from build123d import *

# Parameters (mm, degrees)
F1_DEPTH = 8.5


# Not quite as in the source:
# - a feature names something its author has since deleted; it is built from what else it names


with BuildPart() as f1:
    # F0 (on Top) → F1 (new body)
    with BuildSketch(Plane.XY):
        with BuildLine():
            ThreePointArc((-9.25, -7.6444424257), (-11.6891485981, -2.7136331829), (-11.6717637121, 2.7874597484))
            ThreePointArc((-11.6717637121, 2.7874597484), (-11.2656904289, 4.1333060811), (-10.7050113586, 5.42242859))
            Line((-10.7050113586, 5.42242859), (-5.8459149373, 18.8072078091))
            ThreePointArc((-5.8459149373, 18.8072078091), (0, 22.4041745059), (5.8459149373, 18.8072078091))
            Line((5.8459149373, 18.8072078091), (10.7050113586, 5.42242859))
            ThreePointArc((10.7050113586, 5.42242859), (11.2656904289, 4.1333060811), (11.6717637121, 2.7874597484))
            ThreePointArc((11.6717637121, 2.7874597484), (11.6891485981, -2.7136331829), (9.25, -7.6444424257))
            Line((9.25, -7.6444424257), (9.25, -11.1663557171))
            Line((9.25, -11.1663557171), (9.25, -20.1444424257))
            Line((9.25, -20.1444424257), (3.25, -20.1444424257))
            Line((3.25, -20.1444424257), (3.25, -21.1444424257))
            Line((3.25, -21.1444424257), (3.25, -23.6444424257))
            Line((3.25, -23.6444424257), (7, -26.1444424257))
            Line((7, -26.1444424257), (9.25, -26.1444424257))
            Line((9.25, -26.1444424257), (9.25, -27.6444424257))
            Line((9.25, -27.6444424257), (14.25, -27.6444424257))
            Line((14.25, -27.6444424257), (14.25, -21.4303609628))
            Line((14.25, -21.4303609628), (14.25, -2.6809513237))
            ThreePointArc((14.25, -2.6809513237), (14.437364718, -1.3462912018), (14.5, 0))
            ThreePointArc((14.5, 0), (14.400503927, 1.6957259941), (14.1033811521, 3.3681805293))
            ThreePointArc((14.1033811521, 3.3681805293), (13.8091695526, 4.4223111907), (13.4362898945, 5.4512488358))
            Line((13.4362898945, 5.4512488358), (8.4985279846, 18.8072078091))
            ThreePointArc((8.4985279846, 18.8072078091), (0, 24.7259901099), (-8.4985279846, 18.8072078091))
            Line((-8.4985279846, 18.8072078091), (-13.4362898945, 5.4512488358))
            ThreePointArc((-13.4362898945, 5.4512488358), (-13.8091695526, 4.4223111907), (-14.1033811521, 3.3681805293))
            ThreePointArc((-14.1033811521, 3.3681805293), (-14.400503927, 1.6957259941), (-14.5, 0))
            ThreePointArc((-14.5, 0), (-14.437364718, -1.3462912018), (-14.25, -2.6809513237))
            Line((-14.25, -2.6809513237), (-14.25, -21.1444424257))
            Line((-14.25, -21.1444424257), (-14.25, -27.6444424257))
            Line((-14.25, -27.6444424257), (-9.25, -27.6444424257))
            Line((-9.25, -27.6444424257), (-9.25, -26.1444424257))
            Line((-9.25, -26.1444424257), (-7, -26.1444424257))
            Line((-7, -26.1444424257), (-3.25, -23.6444424257))
            Line((-3.25, -23.6444424257), (-3.25, -21.1444424257))
            Line((-3.25, -21.1444424257), (-3.25, -20.1444424257))
            Line((-3.25, -20.1444424257), (-9.25, -20.1444424257))
            Line((-9.25, -20.1444424257), (-9.25, -11.1663557171))
            Line((-9.25, -11.1663557171), (-9.25, -7.6444424257))
        make_face()
    extrude(amount=-F1_DEPTH)


solid = f1.part
Verification items for the finished model (mm, model axes). A direction names the side the tool comes from. Give positions to 0.01 mm unless a question says otherwise; leave off trailing zeros. Order: outer loops, then holes, each group sorted by start corner. A loop starts at its lowest first (then second) coordinate and runs counter-clockwise, first axis right, second up. Notation, with made-up numbers: M 5.5,78 L 9.5,78 A21 cw 9.5,99 Z; hole C 82,7.5 d8. An arc over 180 degrees is marked long. Use one line per item in the form item = value. Start each with the question number.
Q1. Section check C-C (x = -4). Enter the section's corners in (y, z).
Q2. Mould release check, pull along X, two halves, no side actions. Record for faces 4 (the cylindrical face through (0.154, 24.725, -4.19)), 5 (the flat face through (14.25, -15, -4)), 6 (the flat face through (5.1, -24.88, -4.19)): +X half, -X half, draft (parallel to the pull), parting line (faces both ways), or undercut.
Q3. Scan lines: line 1 along X through (y, z) = (-14, -4.25); line 2 along X through (y, z) = (-23.5, -7.25); line 3 along Y through (x, z) = (4, -4.25). Record each from-to range of solid material in increasing order. Write a range as [from, to].
Q4. Section check A-A (y = -12.5). Enter the section's corners in (x, z), then the cut area to 3 significant figures.
Q5. Access from +Z, -Z, +X, -X, +Y, -Y to the whole of each face (thin tool, end or side, straight path). Record for faces 1 (the flat face through (-14.25, -15, -4)), 2 (the flat face through (-9.25, -14, -4)), 3 (the flat face through (-8, -26.144, -4)).
Q6. Section check B-B (z = -7). Enter the section's corners in (x, y).
Q7. Go/stop test with flat-tipped pins: pin 1 Ø4 at (y, z) = (-21.5, -5) entering from -X; pin 2 Ø5 at (x, z) = (-5, -3.5) entering from +Y; pin 3 Ø1 at (x, z) = (-1, -5) entering from +Y; pin 4 Ø6 at (x, y) = (6.5, -18.5) entering from +Z. Record where each tip stops, or that it passes through.
Q8. Section check D-D (x = -0.75). Enter the section's corners in (y, z), then the cut area to 3 significant figures.
Evaluation:
q1.outline = M -24.14,-8.5 L -20.14,-8.5 L -20.14,0 L -24.14,0 Z; M 21.04,-8.5 L 23.8,-8.5 L 23.8,0 L 21.04,0 Z
q2.face_4 = parting line
q2.face_5 = +X half
q2.face_6 = undercut
q3.line_1 = [-14.25, -9.25], [9.25, 14.25]
q3.line_2 = [-14.25, -3.25], [3.25, 14.25]
q3.line_3 = [-24.14, -20.14], [21.04, 23.8]
q4.outline = M -14.25,-8.5 L -9.25,-8.5 L -9.25,0 L -14.25,0 Z; M 9.25,-8.5 L 14.25,-8.5 L 14.25,0 L 9.25,0 Z
q4.area = 85.0 mm2
q5.face_1 = +Z, -Z, -X, -Y
q5.face_2 = +Z, -Z
q5.face_3 = +Z, -Z, -Y
q6.outline = M -14.25,-27.64 L -9.25,-27.64 L -9.25,-26.14 L -7,-26.14 L -3.25,-23.64 L -3.25,-20.14 L -9.25,-20.14 L -9.25,-7.64 A12 cw -10.71,5.42 L -5.85,18.81 A6.55 cw 5.85,18.81 L 10.71,5.42 A12 cw 9.25,-7.64 L 9.25,-20.14 L 3.25,-20.14 L 3.25,-23.64 L 7,-26.14 L 9.25,-26.14 L 9.25,-27.64 L 14.25,-27.64 L 14.25,-2.68 A14.5 ccw 13.44,5.45 L 8.5,18.81 A9.06 ccw -8.5,18.81 L -13.44,5.45 A14.5 ccw -14.25,-2.68 Z
q7.pin_1 = -14.25
q7.pin_2 = 24.37
q7.pin_3 = 24.71
q7.pin_4 = 0
q8.outline = M 22.36,-8.5 L 24.69,-8.5 L 24.69,0 L 22.36,0 Z
q8.area = 19.8 mm2
